```python
from build123d import *

# Parameters (mm, degrees)
F1_DEPTH = 12
F3_DEPTH = 43.501
F4_R     = 2
F5_DEPTH = 12.001
F6_R     = 4
F7_DEPTH = 1
F8_SIZE  = 1.6


with BuildPart() as f1:
    # F0 (on Top) → F1 (new body)
    with BuildSketch(Plane.XY):
        with BuildLine():
            Line((-5, 32.5), (-30, 32.5))
            Line((-30, 32.5), (-30, -32.5))
            Line((-30, -32.5), (-20, -32.5))
            Line((-20, -32.5), (-20, -12.24))
            Line((-20, -12.24), (-3, -32.5))
            Line((-3, -32.5), (12, -32.5))
            Line((12, -32.5), (-11.494571, -4.5))
            Line((-11.494571, -4.5), (-5, -4.5))
            ThreePointArc((-5, -4.5), (13.5, 14), (-5, 32.5))
        make_face()
        with BuildLine():
            Line((-18, 6.5), (-18, 21.5))
            Line((-18, 21.5), (-6, 21.5))
            ThreePointArc((-6, 21.5), (1.5, 14), (-6, 6.5))
            Line((-6, 6.5), (-18, 6.5))
        make_face(mode=Mode.SUBTRACT)
    extrude(amount=F1_DEPTH)

    # F2 (on face) → F3 (cut, through all)
    with BuildSketch(Plane(origin=(-30, 0, 0), x_dir=(0, -1, 0), z_dir=(-1, 0, 0))):
        with BuildLine():
            Line((32.5, 11), (30.5, 11))
            ThreePointArc((30.5, 11), (25.5, 6), (30.5, 1))
            Line((30.5, 1), (32.5, 1))
            Line((32.5, 1), (32.5, 11))
        make_face()
    extrude(amount=-F3_DEPTH, mode=Mode.SUBTRACT)

    # F4 (on face) → F5 (cut, through all)
    with BuildSketch(Plane.XY.offset(12)):
        with Locations((-20, 1.5)):
            Circle(F4_R)
    extrude(amount=-F5_DEPTH, mode=Mode.SUBTRACT)

    # F6 (on face) → F7 (cut)
    with BuildSketch(Plane.XY.offset(12)):
        with Locations((-20, 1.5)):
            Circle(F6_R)
    extrude(amount=-F7_DEPTH, mode=Mode.SUBTRACT)

    # F8
    f8_edges = [f1.edges().sort_by_distance(p)[0] for p in [
        (-22, 1.5, 11),
    ]]
    chamfer(f8_edges, length=F8_SIZE)


solid = f1.part
```
Work out the finished part from the listing and answer in its coordinate system (mm). A direction names the side the tool comes from. Give positions to 0.01 mm unless a question says otherwise; leave off trailing zeros. Loops run counter-clockwise (first coordinate to the right, second up) from the corner with the lowest first, then second, coordinate; pieces in that order, holes last. Notation, with made-up numbers: (-14, -38.5) -> (41, -38.5) arc R31 ccw to (41, -3.5) -> close; hole circle Ø2 at (56.25, 88.5). An arc over 180 degrees is marked (long way). One line per question, with ' | ' between items. Start each with the question number.
1) Determine the mould class of faces 1 (the face through (-20, -20, 6)), 2 (the face through (-2.193, -15.585, 5.916)), 3 (the face through (-12, 6.5, 6)), 4 (the face through (-25, -31, 1)) for opening direction X: +X half, -X half, draft (parallel to the pull), parting line (faces both ways), or undercut.
2) Straight lines are drawn through the part: L1, parallel to Y at x = -6.5, z = 9.25; L2, parallel to Y at x = -13.5, z = 11; L3, parallel to Y at x = -10.5, z = 4. For each, find the intervals that lie inside material, in ascending order.
3) Section D-D, the plane x = -26 is taken. Determine the outline of the cut face in (y, z), then the cut area to 3 significant figures.
4) Section B-B, the plane x = 5 is taken. Determine the outline of the cut face in (y, z).
5) Each of these flat-tipped pins is pushed along its axis until it touches: pin 1 (5 mm diameter, centred on x = -20, y = 1.5, fed in from +Z); pin 2 (1.9 mm diameter, centred on x = -8.5, z = 7.5, fed in from -Y); pin 3 (6 mm diameter, centred on x = -13.5, z = 4.5, fed in from -Y); pin 4 (1 mm diameter, centred on x = 4, y = -31.5, fed in from -Z). Where does it stop, or does it pass through?
6) Section A-A, the plane y = 14 is taken. Determine the outline of the cut face in (x, z), then the cut area to 3 significant figures.
7) For faces 5 (the face through (-23.2, -0.9, 11.5)), 6 (the face through (4, -32, 11)), 7 (the face through (-13.508, -19.977, 5.916)), 8 (the face through (-12, 21.5, 6)), determine the directions among +Z, -Z, +X, -X, +Y, -Y from which every point of the face is accessible in a straight line to the end or side of a thin tool.
8) Section C-C, the plane z = 7.5 is taken. Determine the outline of the cut face in (x, y), then the cut area to 3 significant figures.
Resolved:
1) face 1: undercut | face 2: +X half | face 3: undercut | face 4: draft
2) L1: -26.7 to -10.45, -4.5 to 6.5, 21.5 to 32.5 | L2: -19.99 to 6.5, 21.5 to 32.5 | L3: -23.56 to -5.69, -4.5 to 6.5, 21.5 to 32.5
3) outline: (-32.5, 0) -> (32.5, 0) -> (32.5, 12) -> (-32.5, 12) -> (-32.5, 11) -> (-30.5, 11) arc R5 cw to (-30.5, 1) -> (-32.5, 1) -> close | area: 721 mm2
4) outline: (-32.5, 0) -> (-24.16, 0) -> (-24.16, 12) -> (-32.5, 12) -> (-32.5, 11) -> (-30.5, 11) arc R5 cw to (-30.5, 1) -> (-32.5, 1) -> close; (-1.56, 0) -> (29.56, 0) -> (29.56, 12) -> (-1.56, 12) -> close
5) pin 1: z = 9.9 | pin 2: y = -26.13 | pin 3: y = -23.56 | pin 4: z = 0
6) outline: (-30, 0) -> (-18, 0) -> (-18, 12) -> (-30, 12) -> close; (1.5, 0) -> (13.5, 0) -> (13.5, 12) -> (1.5, 12) -> close | area: 288 mm2
7) face 5: +Z | face 6: +X, -X, -Y | face 7: +Z, -Z, -Y | face 8: +Z, -Z
8) outline: (-30, -25.73) -> (-20, -25.73) -> (-20, -12.24) -> (-8.68, -25.73) -> (6.32, -25.73) -> (-11.49, -4.5) -> (-5, -4.5) arc R18.5 ccw to (-5, 32.5) -> (-30, 32.5) -> close; hole circle Ø4 at (-20, 1.5); hole (-18, 6.5) -> (-6, 6.5) arc R7.5 ccw to (-6, 21.5) -> (-18, 21.5) -> close | area: 1,690 mm2
